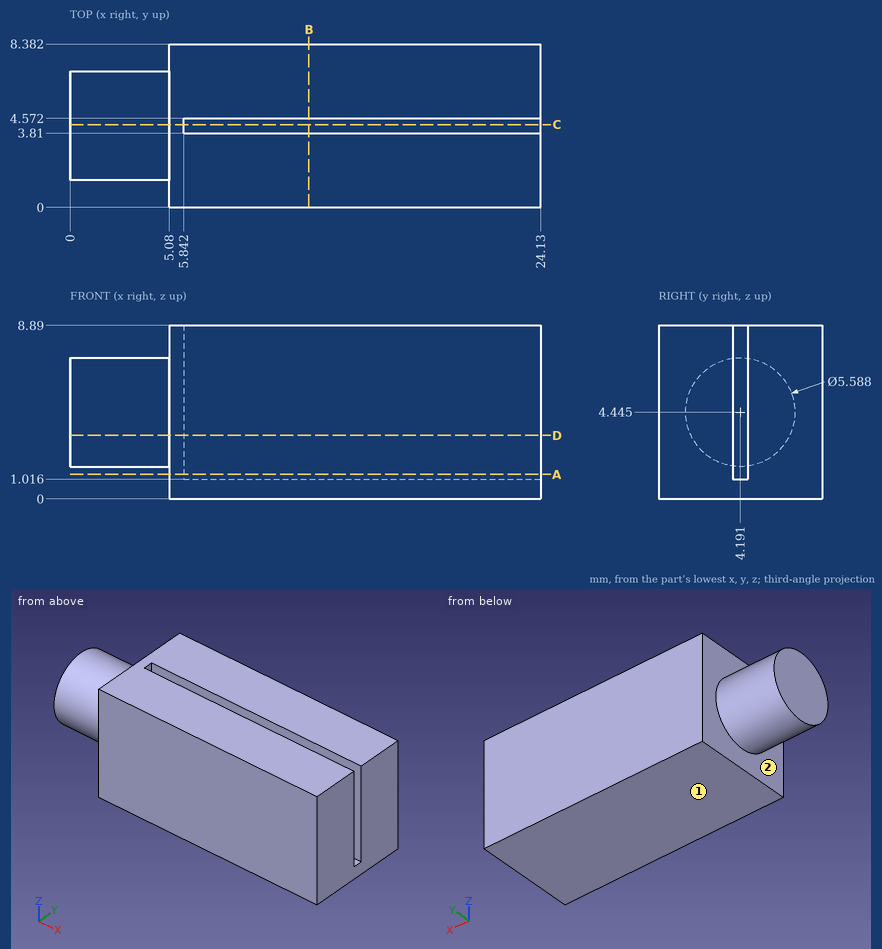
Can you work these out from the drawing? Everything is in mm from the part's minimum corner. A direction names the side the tool comes from. Round coordinates to 2 decimals unless told otherwise and drop trailing zeros. Loops run counter-clockwise (first coordinate to the right, second up) from the corner with the lowest first, then second, coordinate; pieces in that order, holes last. Notation, with made-up numbers: (53, 85.25) - (57, 85.25) arc R15 cw to (57, 93.25) - close; hole circle Ø4 at (-29.75, -26.5). An arc over 180 degrees is marked (long way). Write item = value, one per line. Start each with the question number.
(1) For the marked faces 1 and 2, which set-ups out of +Z, -Z, +X, -X, +Y, -Y let a thin tool reach every point of the face, with its end or its side?
(2) If we section it at B-B (x = 12.25): Please give me the cut outline in (y, z), and give its area (3 significant figures).
(3) If I drill on probe 1 along Y at (x, z) = (22, 3.25); probe 2 along X at (y, z) = (6, 8.5); probe 3 along Z at (x, y) = (1.75, 4.25), over which ranges is the centre line in solid material (lowest first)? Write a range as [from, to].
(4) If we section it at C-C (y = 4.25): Please give me the cut outline in (x, z).
(5) If we section it at A-A (z = 1.25): Please give me the cut outline in (x, y).
(6) If we section it at D-D (z = 3.25): Please give me the cut outline in (x, y).
Ans:
q1.face_1 = -Z, +X, -X, +Y, -Y
q1.face_2 = -X
q2.outline = (0, 0) - (8.38, 0) - (8.38, 8.89) - (4.57, 8.89) - (4.57, 1.02) - (3.81, 1.02) - (3.81, 8.89) - (0, 8.89) - close
q2.area = 68.5 mm²
q3.probe_1 = [0, 3.81], [4.57, 8.38]
q3.probe_2 = [5.08, 24.13]
q3.probe_3 = [1.65, 7.24]
q4.outline = (0, 1.65) - (5.08, 1.65) - (5.08, 0) - (24.13, 0) - (24.13, 1.02) - (5.84, 1.02) - (5.84, 8.89) - (5.08, 8.89) - (5.08, 7.24) - (0, 7.24) - close
q5.outline = (5.08, 0) - (24.13, 0) - (24.13, 3.81) - (5.84, 3.81) - (5.84, 4.57) - (24.13, 4.57) - (24.13, 8.38) - (5.08, 8.38) - close
q6.outline = (0, 1.67) - (5.08, 1.67) - (5.08, 0) - (24.13, 0) - (24.13, 3.81) - (5.84, 3.81) - (5.84, 4.57) - (24.13, 4.57) - (24.13, 8.38) - (5.08, 8.38) - (5.08, 6.72) - (0, 6.72) - close
